Here's how the part is built. I have some questions about the finished solid (model axes, mm). A direction names the side the tool comes from. Coordinates: 2 decimals unless noted, no trailing zeros. Write each loop counter-clockwise with the first axis right and the second up, starting at its lowest first coordinate (ties: lowest second). Pieces come first, ordered by that corner, then holes.
(1) Please list where these lines run through material, in increasing order: probe 1 along Z at (x, y) = (19, 15) (3 decimals); probe 2 along Y at (x, z) = (29.9, 2.3); probe 3 along Z at (x, y) = (8.5, 26.25) (3 decimals).
(2) Imagine slicing it at C-C, the plane x = 51. List the corners of the cut face in (y, z) for me (3 decimals).
(3) Imagine slicing it at D-D, the plane x = 29.9. List the corners of the cut face in (y, z) for me (3 decimals), plus the area to 3 significant figures.
(4) Imagine slicing it at B-B, the plane z = 5.05. List the corners of the cut face in (x, y) for me (3 decimals).
(5) For pin 1 Ø5 at (x, z) = (19, 5.05) entering from -Y; pin 2 Ø3.5 at (x, y) = (29.9, 19.175) entering from -Z; pin 3 Ø6.5 at (x, y) = (80, 9.175) entering from -Z (3 decimals); pin 4 Ø10 at (y, z) = (10.5, 8.5) entering from -X, each with a flat end and sliding along its axis, tell me the tip position at first contact or that it passes through.
(6) Which directions (+Z, -Z, +X, -X, +Y, -Y) give clear straight access to the entire face, cutting with the end or side of a thin tool? Please do faces 1 (the flat face through (7, 14, 20.1)), 2 (the cylindrical face through (17.23, 13.98, 13.92)), 3 (the flat face through (75, 14, 3)).
(7) Thinking about a two-plate mould opening in Z: for faces 4 (the flat face through (0, 14, 22)), 5 (the flat face through (14, 14, 10)), 6 (the flat face through (47, 27, 0.825)), which applies, released by +Z, released by -Z, zero draft, split by the parting line, or undercut?
(8) Imagine slicing it at A-A, the plane y = 12.25. List the corners of the cut face in (x, z) for me (3 decimals).
```python
from build123d import *

# Parameters (mm, degrees)
SKETCH1_R               = 2.1
BOSS_EXTRUDE1_DEPTH     = 28.35
SKETCH2_W               = 5
SKETCH2_H               = 28.35
BOSS_EXTRUDE2_DEPTH     = 58
CUT_EXTRUDE1_DEPTH      = 91.535766413
CUT_EXTRUDE1_DEPTH_BACK = 91.535766413
SKETCH3_W               = 40.1
SKETCH3_H               = 20.1
CUT_EXTRUDE2_DEPTH      = 91.535766413
CUT_EXTRUDE2_DEPTH_BACK = 91.535766413
SKETCH4_R               = 2.075
FILLET1_R               = 6


with BuildPart() as part:
    # Sketch1 → Boss-Extrude1 (new body)
    with BuildSketch(Plane(origin=(0, 0, 0), x_dir=(1, 0, 0), z_dir=(0, 1, 0))):
        Polygon((0, 0), (14, 0), (14, -20.1), (0, -20.1), (0, -23.275), (25, -23.275), (25, 3.175), (0, 3.175), align=None)
        with Locations(Location((19, -5.05, 0), (0, 0, 90))):
            Circle(SKETCH1_R, mode=Mode.SUBTRACT)
        with Locations(Location((19, -15.05, 0), (0, 0, 90))):
            Circle(SKETCH1_R, mode=Mode.SUBTRACT)
    extrude(amount=BOSS_EXTRUDE1_DEPTH)

    # Sketch2 → Boss-Extrude2 (add)
    with BuildSketch(Plane(origin=(25, 0, 0), x_dir=(0, 0, -1), z_dir=(1, 0, 0))):
        with Locations((-3.325, 14.175)):
            Rectangle(SKETCH2_W, SKETCH2_H)
    extrude(amount=BOSS_EXTRUDE2_DEPTH)

    # Sketch3 → Cut-Extrude1 (cut, two sides: drawn at the far end of the back side and taken through both)
    with BuildSketch(Plane(origin=(0, 0, 0.825), x_dir=(-1, 0, 0), z_dir=(0, 0, -1)).offset(-CUT_EXTRUDE1_DEPTH_BACK)):
        with Locations((-54.95, 14.175)):
            Rectangle(SKETCH3_W, SKETCH3_H)
    extrude(amount=CUT_EXTRUDE1_DEPTH + CUT_EXTRUDE1_DEPTH_BACK, mode=Mode.SUBTRACT)

    # Sketch4 → Cut-Extrude2 (cut, two sides: drawn at the far end of the back side and taken through both)
    with BuildSketch(Plane(origin=(0, 0, 0.825), x_dir=(-1, 0, 0), z_dir=(0, 0, -1)).offset(-CUT_EXTRUDE2_DEPTH_BACK)):
        with Locations(Location((-29.9, 19.175, 0), (0, 0, 90))):
            Circle(SKETCH4_R)
        with Locations(Location((-29.9, 9.175, 0), (0, 0, 90))):
            Circle(SKETCH4_R)
        with Locations(Location((-80, 19.175, 0), (0, 0, 90))):
            Circle(SKETCH4_R)
        with Locations(Location((-80, 9.175, 0), (0, 0, 90))):
            Circle(SKETCH4_R)
    extrude(amount=CUT_EXTRUDE2_DEPTH + CUT_EXTRUDE2_DEPTH_BACK, mode=Mode.SUBTRACT)

    # Fillet1
    # the kernel refuses this fillet: 6 mm, written as the material it takes off along each edge
    with BuildSketch(Plane(origin=(25, -14.142135624, -3.175), x_dir=(-1, 0, 0), z_dir=(0, 1, 0))) as fillet1_piece_1:
        with BuildLine():
            CenterArc((5.656854249, 6), FILLET1_R, 199.471220634, 70.528779366)
            Line((0, 4), (-0.113137085, 3.96))
            ThreePointArc((-0.113137085, 3.96), (-0.12, 2), (-0.12, 0))
            Line((-0.12, 0), (0, -0.12))
            Line((0, -0.12), (5.656854249, -0.12))
            Line((5.656854249, -0.12), (5.656854249, 0))
        make_face()
    extrude(amount=56.634271247, mode=Mode.SUBTRACT)
    with BuildSketch(Plane(origin=(25, -15, 23.275), x_dir=(-1, 0, 0), z_dir=(0, 1, 0))) as fillet1_piece_2:
        with BuildLine():
            CenterArc((FILLET1_R, -FILLET1_R), FILLET1_R, 90, 90)
            Line((0, -FILLET1_R), (-FILLET1_R * 0.02, -FILLET1_R))
            Line((-FILLET1_R * 0.02, -FILLET1_R), (-FILLET1_R * 0.02, FILLET1_R * 0.02))
            Line((-FILLET1_R * 0.02, FILLET1_R * 0.02), (FILLET1_R, FILLET1_R * 0.02))
            Line((FILLET1_R, FILLET1_R * 0.02), (FILLET1_R, 0))
        make_face()
    extrude(amount=58.35, mode=Mode.SUBTRACT)


solid = part.part
```
Recorded:
1. probe 1: z = -3.175 to 2.95, 7.15 to 12.95, 17.15 to 23.275
1. probe 2: y = 0 to 7.1, 11.25 to 17.1, 21.25 to 28.35
1. probe 3: z = -3.175 to 0, 20.1 to 23.275
2. outline: (0, 0.825) - (4.125, 0.825) - (4.125, 5.825) - (0, 5.825) - close; (24.225, 0.825) - (28.35, 0.825) - (28.35, 5.825) - (24.225, 5.825) - close
3. outline: (0, 0.825) - (7.1, 0.825) - (7.1, 5.825) - (0, 5.825) - close; (11.25, 0.825) - (17.1, 0.825) - (17.1, 5.825) - (11.25, 5.825) - close; (21.25, 0.825) - (28.35, 0.825) - (28.35, 5.825) - (21.25, 5.825) - close
3. area: 100 mm2
4. outline: (14, 0) - (16.9, 0) - (16.9, 28.35) - (14, 28.35) - close; (21.1, 0) - (83, 0) - (83, 28.35) - (21.1, 28.35) - close; hole circle Ø4.15 at (29.9, 9.175); hole circle Ø4.15 at (29.9, 19.175); hole (34.9, 4.125) - (75, 4.125) - (75, 24.225) - (34.9, 24.225) - close; hole circle Ø4.15 at (80, 9.175); hole circle Ø4.15 at (80, 19.175)
5. pin 1: stops at y = 0
5. pin 2: passes through
5. pin 3: stops at z = 0.825
5. pin 4: stops at x = 14
6. face 1: -X, +Y, -Y
6. face 2: +Y, -Y
6. face 3: +Z, -Z
7. face 4: zero draft
7. face 5: undercut
7. face 6: released by -Z
8. outline: (0, -3.175) - (19.343, -3.175) arc R6 ccw to (25, 0.825) - (34.9, 0.825) - (34.9, 5.825) - (25, 5.825) - (25, 17.275) arc R6 ccw to (19, 23.275) - (0, 23.275) - (0, 20.1) - (14, 20.1) - (14, 0) - (0, 0) - close; (75, 0.825) - (83, 0.825) - (83, 5.825) - (75, 5.825) - close; hole circle Ø4.2 at (19, 5.05); hole circle Ø4.2 at (19, 15.05)
